Input: part model. Units: mm. Frame: model coordinates. A direction names the side the tool comes from. Give positions to 0.01 mm unless a question says otherwise; leave off trailing zeros. Order: outer loops, then holes, each group sorted by start corner. A loop starts at its lowest first (then second) coordinate and runs counter-clockwise, first axis right, second up. Notation, with made-up numbers: M -38.75,78 L 3.25,78 A6 ccw 3.25,84 Z; hole C 25,34.25 d7. An arc over 180 degrees is marked long. Use a Markdown table: item, result.
Autodesk Inventor part; units mm, degrees
ref_plane "YZ Plane" through (0, 0, 0) normal (1, 0, 0) x (0, 1, 0)
ref_plane "XZ Plane" through (0, 0, 0) normal (0, 1, 0) x (-1, 0, 0)
ref_plane "XY Plane" through (0, 0, 0) normal (0, 0, 1) x (1, 0, 0)
sketch "Sketch1" plane through (0, 0, 0) normal (0, 0, 1) x (1, 0, 0)
  circle A0 centre (0, 0) radius 10
  circle A1 centre (0, 0) radius 20
  line L0 (-15, 0) -> (15, 0)
  line L1 (15, 0) -> (15, 50)
  line L2 (15, 50) -> (-15, 50)
  line L3 (-15, 50) -> (-15, 0)
  point P0 (-15, 13.2288)
  point P1 (15, 13.2288)
  dimension "d0" = 20
  dimension "d1" = 40
  dimension "d2" = 30
  dimension "d3" = 50
extrude "Extrusion1" add sketch "Sketch1" along normal blind 20
sketch "Sketch2" plane through (0, 0, 20) normal (0, 0, 1) x (1, 0, 0)
  circle A0 centre (0, 0) radius 10
  dimension "d6" = 20
extrude "Extrusion2" cut sketch "Sketch2" against normal blind 15
sketch "Sketch4" plane through (-15, 13.2288, 0) normal (-1, 0, 0) x (0, 0, 1)
  line L0 (0, 36.7712) -> (20, 36.7712)
  line L1 (0, 0) -> (0, 36.7712)
  line L2 (20, 36.7712) -> (0, 36.7712)
  line L3 (0, 36.7712) -> (0, 0)
  line L4 (0, 0) -> (20, 0)
  line L5 (20, 0) -> (20, 36.7712)
  line L6 (0, 0) -> (20, 0)
  line L7 (20, 36.7712) -> (10, 36.7712)
  line L8 (10, 36.7712) -> (10, 0)
  line L9 (10, 0) -> (20, 0)
  line L10 (20, 0) -> (20, 36.7712)
  line L11 (10, 0) -> (16, 0)
  line L12 (16, 0) -> (16, 25)
  line L13 (16, 25) -> (10, 25)
  line L14 (10, 25) -> (10, 0)
  line L15 (10, 25) -> (4, 25)
  line L16 (4, 25) -> (4, 0)
  line L17 (4, 0) -> (10, 0)
  line L18 (10, 0) -> (10, 25)
  line L19 (4, 25) -> (16, 25)
  line L20 (16, 25) -> (16, 30.0005)
  line L21 (16, 30.0005) -> (4, 30.0005)
  line L22 (4, 30.0005) -> (4, 25)
  line L23 (4, 30.0005) -> (16, 30.0005)
  line L24 (16, 30.0005) -> (16, 7.0005)
  line L25 (16, 7.0005) -> (4, 7.0005)
  line L26 (4, 7.0005) -> (4, 30.0005)
  line L27 (10, 7.0005) -> (16, 7.0005)
  line L28 (16, 7.0005) -> (16, 0)
  line L29 (16, 0) -> (10, 0)
  line L30 (10, 0) -> (10, 7.0005)
  point P0 (0, -13.2288)
  dimension "d13" = 6
  dimension "d14" = 25
  dimension "d15" = 6
  dimension "d16" = 23
extrude "Extrusion3" cut sketch "Sketch4" against normal blind 23 contours L21 L20 L13 L8 | L8 L15 L22 L21 | L13 L12 L25 L8 | L8 L25 L16 L15
sketch "Sketch6" plane through (-15, 13.2288, 0) normal (-1, 0, 0) x (0, 0, 1)
  line L0 (4, 7.0005) -> (4, 30.0005)
  line L1 (4, 7.0005) -> (16, 7.0005)
  line L2 (16, 7.0005) -> (16, 2.2005)
  line L3 (16, 2.2005) -> (4, 2.2005)
  line L4 (4, 2.2005) -> (4, 7.0005)
  line L5 (4, 30.0005) -> (16, 30.0005)
  line L6 (16, 30.0005) -> (16, 34.8005)
  line L7 (16, 34.8005) -> (4, 34.8005)
  line L8 (4, 34.8005) -> (4, 30.0005)
  point P0 (0, -13.2288)
  dimension "d19" = 12
  dimension "d20" = 4.8
  dimension "d21" = 4.8
extrude "Extrusion4" cut sketch "Sketch6" against normal blind 16
sketch "Sketch7" plane through (1, 13.2288, 0) normal (-1, 0, 0) x (0, 0, 1)
  line L0 (4, 30.0005) -> (16, 30.0005)
  line L1 (4, 30.0005) -> (10, 30.0005)
  line L2 (10, 30.0005) -> (10, 32.5005)
  line L3 (10, 32.5005) -> (4, 32.5005)
  line L4 (4, 32.5005) -> (4, 30.0005)
  circle A0 centre (10, 32.5005) radius 0.75
  line L5 (16, 7.0005) -> (4, 7.0005)
  line L6 (16, 7.0005) -> (16, 2.2005)
  line L7 (4, 7.0005) -> (16, 7.0005)
  line L8 (16, 7.0005) -> (16, 4.5005)
  line L9 (16, 4.5005) -> (4, 4.5005)
  line L10 (4, 4.5005) -> (4, 7.0005)
  line L11 (10, 4.5005) -> (4, 4.5005)
  line L12 (4, 4.5005) -> (4, 7.0005)
  line L13 (4, 7.0005) -> (10, 7.0005)
  line L14 (10, 7.0005) -> (10, 4.5005)
  circle A1 centre (10, 4.5005) radius 0.75
  point P0 (0, -13.2288)
  dimension "d24" = 2.5
  dimension "d25" = 1.5
  dimension "d26" = 2.5
  dimension "d27" = 1.5
extrude "Extrusion5" cut sketch "Sketch7" against normal blind 8 contours A0 L3 L2 | L2 L3 A0 | A1 L9 L14 | L14 L9 A1 | A1 L9
sketch "Sketch8" plane through (15, 13.2288, 0) normal (1, 0, 0) x (0, 0, -1)
  line L0 (0, 36.7712) -> (0, 0)
  line L1 (-20, 36.7712) -> (-20, 0)
  line L2 (0, 36.7712) -> (-20, 36.7712)
  line L3 (-20, 36.7712) -> (-20, 26.7712)
  line L4 (-20, 26.7712) -> (0, 26.7712)
  line L5 (0, 26.7712) -> (0, 36.7712)
  line L6 (0, 26.7712) -> (-20, 26.7712)
  line L7 (-20, 26.7712) -> (-20, 18.7712)
  line L8 (-20, 18.7712) -> (0, 18.7712)
  line L9 (0, 18.7712) -> (0, 26.7712)
  line L10 (0, 26.7712) -> (-10, 26.7712)
  line L11 (-10, 26.7712) -> (-10, 18.7712)
  line L12 (-10, 18.7712) -> (0, 18.7712)
  line L13 (0, 18.7712) -> (0, 26.7712)
  line L14 (-10, 26.7712) -> (-5, 26.7712)
  line L15 (-5, 26.7712) -> (-5, 22.7712)
  line L16 (-5, 22.7712) -> (-10, 22.7712)
  line L17 (-10, 22.7712) -> (-10, 26.7712)
  line L18 (-10, 22.7712) -> (-15, 22.7712)
  line L19 (-15, 22.7712) -> (-15, 26.7712)
  line L20 (-15, 26.7712) -> (-10, 26.7712)
  line L21 (-10, 26.7712) -> (-10, 22.7712)
  point P0 (0, -13.2288)
  dimension "d30" = 10
  dimension "d31" = 8
  dimension "d32" = 5
  dimension "d33" = 5
extrude "Extrusion6" cut sketch "Sketch8" against normal blind 15.8125 contours L15 L16 L11 L4 | L11 L18 L19 L4
sketch "Sketch9" plane through (0, 0, 5) normal (0, 0, 1) x (1, 0, 0)
  circle A0 centre (0, 0) radius 1
  circle A1 centre (7, 0) radius 1.5
  circle A2 centre (0, 0) radius 1.5
  circle A3 centre (-7, 0) radius 1.5
  dimension "d36" = 2
  dimension "d37" = 3
  dimension "d38" = 3
  dimension "d39" = 3
extrude "Extrusion7" cut sketch "Sketch9" against normal blind 8 contours A0 | A1 | A2 | A3
sketch "Sketch10" plane through (-15, 50, 0) normal (0, 1, 0) x (1, 0, 0)
  line L0 (0, 0) -> (0, -20)
  line L1 (0, 0) -> (29.4792, 0)
  line L2 (29.4792, 0) -> (29.4792, -20)
  line L3 (29.4792, -20) -> (0, -20)
  line L4 (0, -20) -> (0, 0)
  point P0 (15, 0)
extrude "Extrusion8" add sketch "Sketch10" along normal blind 10
sketch "Sketch11" plane through (0, 0, 0) normal (0, 0, -1) x (-1, 0, 0)
  line L0 (15, 13.2288) -> (15, 60)
  line L1 (-15, 13.2288) -> (-15, 50)
  line L2 (15, 60) -> (-15, 60)
  line L3 (-15, 60) -> (-15, 45)
  line L4 (-15, 45) -> (15, 45)
  line L5 (15, 45) -> (15, 60)
  line L6 (15, 45) -> (-15, 45)
  line L7 (-15, 45) -> (-15, 35)
  line L8 (-15, 35) -> (15, 35)
  line L9 (15, 35) -> (15, 45)
  point P0 (0, 0)
  dimension "d47" = 15
  dimension "d48" = 10
sketch "Sketch12" plane through (14.4792, 50, 20) normal (1, 0, 0) x (0, 0, -1)
  line L0 (20, 0) -> (20, 10)
  line L1 (0, 0) -> (20, 0)
  line L2 (20, 0) -> (20, 10)
  line L3 (20, 10) -> (0, 10)
  line L4 (0, 10) -> (0, 0)
  point P0 (20, -50)
extrude "Extrusion9" cut sketch "Sketch12" against normal blind 59.6125
sketch "Sketch13" plane through (-15, 50, 0) normal (0, 1, 0) x (1, 0, 0)
  line L0 (30, 0) -> (30, -20)
  line L1 (0, 0) -> (30, 0)
  line L2 (30, 0) -> (30, -20)
  line L3 (30, -20) -> (0, -20)
  line L4 (0, -20) -> (0, 0)
  point P0 (15, 0)
extrude "Extrusion10" add sketch "Sketch13" along normal blind 10
extrude "Extrusion11" add sketch "Sketch11" along normal blind 10
sketch "Sketch15" plane through (0, 0, 20) normal (0, 0, 1) x (1, 0, 0)
  line L0 (-15, 60) -> (15, 60)
  line L1 (-15, 60) -> (0, 60)
  line L2 (0, 60) -> (0, 35)
  line L3 (0, 35) -> (-15, 35)
  line L4 (-15, 35) -> (-15, 60)
  point P0 (0, 0)
  dimension "d56" = 25
extrude "Extrusion12" add sketch "Sketch15" along normal blind 10
sketch "Sketch16" plane through (0, 0, -10) normal (0, 0, -1) x (-1, 0, 0)
  line L0 (-15, 13.2288) -> (-15, 60)
  line L1 (0, 35) -> (15, 35)
  line L2 (-15, 60) -> (0, 60)
  line L3 (0, 60) -> (0, 35)
  line L4 (0, 35) -> (-15, 35)
  line L5 (-15, 35) -> (-15, 60)
  point P0 (0, 0)
extrude "Extrusion13" cut sketch "Sketch16" against normal blind 10
sketch "Sketch17" plane through (-15, 13.2288, 0) normal (-1, 0, 0) x (0, 0, 1)
  line L0 (0, 0) -> (0, 46.7712)
  line L1 (0, 46.7712) -> (10, 46.7712)
  line L2 (10, 46.7712) -> (10, 23.4712)
  line L3 (10, 23.4712) -> (0, 23.4712)
  line L4 (0, 23.4712) -> (0, 46.7712)
  circle A0 centre (10, 23.4712) radius 10
  line L5 (20, 46.7712) -> (30, 46.7712)
  line L6 (20, 0) -> (20, 46.7712)
  line L7 (30, 46.7712) -> (20, 46.7712)
  line L8 (20, 46.7712) -> (20, 36.7712)
  line L9 (20, 36.7712) -> (30, 36.7712)
  line L10 (30, 36.7712) -> (30, 46.7712)
  line L11 (30, 46.7712) -> (24, 46.7712)
  line L12 (24, 46.7712) -> (24, 36.7712)
  line L13 (24, 36.7712) -> (30, 36.7712)
  line L14 (30, 36.7712) -> (30, 46.7712)
  circle A1 centre (24, 36.7712) radius 2
  line L15 (30, 46.7712) -> (-10, 46.7712)
  line L16 (-10, 46.7712) -> (-4, 46.7712)
  line L17 (-4, 46.7712) -> (-4, 36.7712)
  line L18 (-4, 36.7712) -> (-10, 36.7712)
  line L19 (-10, 36.7712) -> (-10, 46.7712)
  circle A2 centre (-4, 36.7712) radius 2
  point P0 (0, -13.2288)
  dimension "d61" = 23.3
  dimension "d62" = 20
  dimension "d63" = 10
  dimension "d64" = 6
  dimension "d65" = 4
  dimension "d66" = 6
  dimension "d67" = 4
extrude "Extrusion14" add sketch "Sketch17" along normal blind 8 contours A2 L18 L17 | L17 L18 A2 | A1 L12 L9 | L9 A1 | L12 A1 L9
sketch "Sketch18" plane through (0, 0, 20) normal (0, 0, 1) x (1, 0, 0)
  circle A0 centre (0, 0) radius 10
extrude "Extrusion15" add sketch "Sketch18" against normal blind 16
sketch "Sketch19" plane through (0, 0, 0) normal (0, 0, -1) x (-1, 0, 0)
  circle A0 centre (0, 0) radius 1.5
  circle A1 centre (0, 0) radius 10
  dimension "d72" = 20
extrude "Extrusion16" cut sketch "Sketch19" against normal blind 16
sketch "Sketch20" plane through (0, 0, 4) normal (0, 0, -1) x (-1, 0, 0)
  circle A0 centre (0, 0) radius 1.5
  circle A1 centre (0, 0) radius 1.5
extrude "Extrusion17" cut sketch "Sketch20" against normal blind 30.0375
sketch "Sketch21" plane through (0, 0, 16) normal (0, 0, -1) x (-1, 0, 0)
  circle A0 centre (5, 0) radius 1
  circle A1 centre (-5, 0) radius 1
  point P0 (0, 0)
  dimension "d77" = 2
  dimension "d78" = 2
extrude "Extrusion18" cut sketch "Sketch21" against normal blind 138.2375
chamfer "Chamfer2" distance 8 angle 45 1 edges at (10, 0, 0)
sketch "Sketch22" plane through (-15, 13.2288, 0) normal (-1, 0, 0) x (0, 0, 1)
  circle A0 centre (-4, 36.7712) radius 2
  circle A1 centre (-4, 36.7712) radius 2
  circle A2 centre (24, 36.7712) radius 2
  circle A3 centre (24, 36.7712) radius 2
  point P0 (0, -13.2288)
sketch "Sketch25" plane through (-15, 13.2288, 0) normal (-1, 0, 0) x (0, 0, 1)
  circle A0 centre (-4, 36.7712) radius 2
  circle A1 centre (-4, 36.7712) radius 8
  arc A2 (7.7087, 23.1005) -> (12.2913, 23.1005) centre (10, 24.1005) ccw
  circle A3 centre (10, 24.1005) radius 8
  circle A4 centre (24, 36.7712) radius 2
  circle A5 centre (24, 36.7712) radius 8
  circle A6 centre (-4, 36.7712) radius 2
  circle A7 centre (24, 36.7712) radius 2
  line L0 (-4, 36.7712) -> (24.7591, 36.7712)
  line L1 (24.7591, 36.7712) -> (24.7591, 61.7712)
  line L2 (24.7591, 61.7712) -> (-4, 61.7712)
  line L3 (-4, 61.7712) -> (-4, 36.7712)
  point P0 (0, -13.2288)
  dimension "d92" = 16
  dimension "d93" = 16
  dimension "d94" = 16
  dimension "d99" = 25
sketch "Sketch29" plane through (-15, 15.4292, 4) normal (0, 0, 1) x (1, 0, 0)
  point P0 (15, -15.4292)
sketch "Sketch30" plane through (-23, 50, -4) normal (-1, 0, 0) x (0, 0, 1)
  circle A0 centre (0, 0) radius 2
  circle A1 centre (28, 0) radius 2
  circle A2 centre (28, 0) radius 2
  point P0 (4, -50)
extrude "Extrusion24" add sketch "Sketch30" along normal blind 8
sketch "Sketch33" plane through (15, 13.2288, 20) normal (1, 0, 0) x (0, 0, -1)
  line L0 (5, 26.7712) -> (5, 22.7712)
  line L1 (5, 26.7712) -> (15, 26.7712)
  line L2 (15, 26.7712) -> (15, 34.7712)
  line L3 (15, 34.7712) -> (5, 34.7712)
  line L4 (5, 34.7712) -> (5, 26.7712)
  point P0 (20, -13.2288)
  dimension "d110" = 10
  dimension "d111" = 8
extrude "Extrusion27" cut sketch "Sketch33" against normal blind 7
sketch "Sketch34" plane through (0, 0, 30) normal (0, 0, 1) x (1, 0, 0)
  point P0 (0, 0)
sketch "Sketch35" plane through (-15, 13.2288, 0) normal (-1, 0, 0) x (0, 0, 1)
  line L0 (0, 46.7712) -> (-10, 46.7712)
  line L1 (-10, 46.7712) -> (4, 46.7712)
  line L2 (4, 46.7712) -> (4, 30.0005)
  line L3 (4, 30.0005) -> (-10, 30.0005)
  line L4 (-10, 30.0005) -> (-10, 46.7712)
  line L5 (30, 46.7712) -> (30, 21.7712)
  line L6 (30, 46.7712) -> (16, 46.7712)
  line L7 (16, 46.7712) -> (16, 30.0005)
  line L8 (16, 30.0005) -> (30, 30.0005)
  line L9 (30, 30.0005) -> (30, 46.7712)
  line L10 (4, 36.7498) -> (16, 36.7498)
  line L11 (16, 36.7498) -> (16, 46.7712)
  line L12 (16, 46.7712) -> (4, 46.7712)
  line L13 (4, 46.7712) -> (4, 36.7498)
  point P0 (0, -13.2288)
extrude "Extrusion28" add sketch "Sketch35" along normal blind 3.5
sketch "Sketch36" plane through (-31, 50, 24) normal (-1, 0, 0) x (0, 0, 1)
  circle A0 centre (-28, 0) radius 2
  circle A1 centre (-28, 0) radius 2
  circle A2 centre (0, 0) radius 2
  point P0 (-24, -50)
extrude "Extrusion29" cut sketch "Sketch36" against normal blind 8
sketch "Sketch37" plane through (0, 0, 30) normal (0, 0, 1) x (1, 0, 0)
  point P0 (0, 0)
sketch "Sketch38" plane through (-15, 13.2288, 0) normal (-1, 0, 0) x (0, 0, 1)
  point P0 (0, -13.2288)
properties part number "EndConnector"
1) Cut plane C-C on x = 5. State how many separate pieces and enclosed holes the cut face has, and give its area (3 significant figures).
Response values:
| item | result |
|---|---|
| separate pieces | 2 |
| enclosed holes | 3 |
| area | 952 mm² |
2) First-contact query: pin 1 Ø4 at (y, z) = (45, 8.5) entering from +X; pin 2 Ø12 at (x, y) = (8, 34) entering from -Z; pin 3 Ø5 at (x, z) = (-9, -5.5) entering from -Y; pin 4 Ø3 at (y, z) = (1, 14) entering from +X. Flat tips, straight axial feed; report the tip coordinate or a pass-through.
Response values:
| item | result |
|---|---|
| pin 1 | stops at x = 8 |
| pin 2 | stops at z = 0 |
| pin 3 | stops at y = 35 |
| pin 4 | stops at x = 20 |
3) Material intervals for line 1 (Y direction, x = 0, z = 14.25); line 2 (Z direction, x = -13, y = 32); line 3 (Y direction, x = 7, z = 10) (3 decimals), sorted ascending. Write a range as from..to.
Response values:
| item | result |
|---|---|
| line 1 | y = -20..-10, 10..15.43, 48.03..60 |
| line 2 | z = 0..4, 16..20 |
| line 3 | y = -18.735..-7.141, 7.141..16.979, 18.479..20.229, 43.229..44.979, 46.479..60 |
4) Cut plane A-A on z = 19. Return loops of the section in (x, y).
Response values:
| item | result |
|---|---|
| outline | M -18.5,43.23 L -15,43.23 L -15,13.23 A20 ccw long 15,13.23 L 15,60 L -18.5,60 Z; hole C -5,0 d2; hole C 0,0 d3; hole C 5,0 d2 |
5) Reachability of faces 1 (the face through (9, 18, 10)), 2 (the face through (-17, 43.229, -3)), 3 (the face through (15, 31, 10)) from +Z, -Z, +X, -X, +Y, -Y: full face, straight path, thin tool, end or side. Return the list, or none.
Response values:
| item | result |
|---|---|
| face 1 | -X |
| face 2 | +Z, -Z, -X |
| face 3 | +Z, -Z, +X, +Y |
6) Mould query, pull axis Z, two halves, no side actions, for faces 4 (the face through (-21, 52, 24)), 5 (the face through (-7, 15.429, 10)), 6 (the face through (-15, 30, 2)). Classes: released by +Z, released by -Z, zero draft, split by the parting line, or undercut.
Response values:
| item | result |
|---|---|
| face 4 | undercut |
| face 5 | undercut |
| face 6 | zero draft |
7) Cut plane B-B on z = -4. Return loops of the section in (x, y), and give its area (3 significant figures).
Response values:
| item | result |
|---|---|
| outline | M -23,48 L -18.5,48 L -18.5,43.23 L -15,43.23 L -15,35 L 0,35 L 0,60 L -18.5,60 L -18.5,52 L -23,52 Z |
| area | 452 mm² |
